The model under review builds one solid part; all positions refer to its coordinate system, in mm. A direction names the side the tool comes from. Round coordinates to 2 decimals unless told otherwise and drop trailing zeros. Loops run counter-clockwise (first coordinate to the right, second up) from the corner with the lowest first, then second, coordinate; pieces in that order, holes last. Notation, with made-up numbers: M 24,11 L 57,11 A25 cw 57,34 Z; hole C 29,83.25 d5. An arc over 180 degrees is marked long. One line per question, with ' | ' between items.
from build123d import *

# Parameters (mm, degrees)
SKETCH3_W                 = 4.35
SKETCH3_H                 = 3.42
SKETCH_PATTERN1_START     = -2.691666667
SKETCH_PATTERN1_OUTLINE_R = 4.35
SKETCH_PATTERN1_DEPTH     = 3.42
SKETCH14_R                = 4.35
CUT_EXTRUDE5_DEPTH        = 0.4275
SKETCH17_OUTSIDE_W        = 88.114
SKETCH17_OUTSIDE_H        = 88.114
SKETCH17_OUTSIDE_R        = 3.768125
CUT_EXTRUDE8_DEPTH        = 9.955029662
CUT_EXTRUDE8_DRAFT        = -75
SKETCH18_OUTSIDE_W        = 82.758
SKETCH18_OUTSIDE_H        = 82.758
SKETCH18_OUTSIDE_R        = 3.768125
CUT_EXTRUDE9_DEPTH        = 9.237544301
CUT_EXTRUDE9_DRAFT        = -75
SKETCH19_OUTSIDE_W        = 93.34
SKETCH19_OUTSIDE_H        = 93.34
SKETCH19_OUTSIDE_R        = 3.768125
CUT_EXTRUDE10_DEPTH       = 10.655226708
CUT_EXTRUDE10_DRAFT       = -75
SKETCH7_R                 = 3
CUT_EXTRUDE1_DEPTH        = 12.317906167
CHAMFER1_SIZE             = 0.158
FILLET2_R                 = 0.1305


# Read off the part's stored shape, not the designer's step: Sketch-Pattern1
with BuildPart() as part:
    # Sketch3 → Revolve1 (revolve)
    with BuildSketch(Plane.XY):
        with Locations((2.175, 3.04)):
            Rectangle(SKETCH3_W, SKETCH3_H)
    revolve(axis=Axis((0, 1.33, 0), (0, 1, 0)))

    # Sketch14 → Cut-Extrude5 (cut)
    with BuildSketch(Plane.XZ.offset(-1.33)):
        Circle(SKETCH14_R)
    extrude(amount=-CUT_EXTRUDE5_DEPTH, mode=Mode.SUBTRACT)


with BuildPart() as body_2:
    # Sketch6 → Revolve2 (revolve)
    with BuildSketch(Plane.XY):
        Polygon((3.7525, 0.728333333), (3.7525, -2.691666667), (3.7525, -3.720833333), (3.95, -3.720833333), (3.95, -4.75), (0, -4.75), (0, 1.7575), (3.7525, 1.7575), align=None)
    revolve(axis=Axis((0, -4.75, 0), (0, 1, 0)))


with BuildPart() as body_3:
    # Sketch-Pattern1 outline → Sketch-Pattern1 (new body)
    with BuildSketch(Plane(origin=(0, 0, 0), x_dir=(1, 0, 0), z_dir=(0, 1, 0)).offset(SKETCH_PATTERN1_START)):
        Circle(SKETCH_PATTERN1_OUTLINE_R)
    extrude(amount=SKETCH_PATTERN1_DEPTH)


with BuildPart() as body_4:
    # Mirror3: mirrored copy
    add(body_3.part.mirror(Plane.XY))


with BuildPart() as cut_extrude8_tool:
    # Sketch17 outside → Cut-Extrude8 (with draft: the straight prism first)
    with BuildSketch(Plane.XZ.offset(-1.7575)):
        Rectangle(SKETCH17_OUTSIDE_W, SKETCH17_OUTSIDE_H)
        Circle(SKETCH17_OUTSIDE_R, mode=Mode.SUBTRACT)
    extrude(amount=-CUT_EXTRUDE8_DEPTH)
    # Cut-Extrude8: the draft: its side faces are tilted about the plane it starts from
    cut_extrude8_sides = [cut_extrude8_tool.faces().sort_by_distance(p)[0] for p in [
        (0, 6.735014831, -44.057),
        (44.057, 6.735014831, 0),
        (0, 6.735014831, 44.057),
        (-44.057, 6.735014831, 0),
        (-3.768125, 6.735014831, 0),
    ]]
    draft(cut_extrude8_sides, Plane.XZ.offset(-1.7575), CUT_EXTRUDE8_DRAFT)


with BuildPart() as part_1:
    add(part.part)

    # Cut-Extrude8: cut by cut_extrude8_tool
    add(cut_extrude8_tool.part, mode=Mode.SUBTRACT)


with BuildPart() as cut_extrude9_tool:
    # Sketch18 outside → Cut-Extrude9 (with draft: the straight prism first)
    with BuildSketch(Plane(origin=(0, 0.728333333, 0), x_dir=(1, 0, 0), z_dir=(0, 1, 0))):
        Rectangle(SKETCH18_OUTSIDE_W, SKETCH18_OUTSIDE_H)
        Circle(SKETCH18_OUTSIDE_R, mode=Mode.SUBTRACT)
    extrude(amount=-CUT_EXTRUDE9_DEPTH)
    # Cut-Extrude9: the draft: its side faces are tilted about the plane it starts from
    cut_extrude9_sides = [cut_extrude9_tool.faces().sort_by_distance(p)[0] for p in [
        (0, -3.890438817, 41.379),
        (41.379, -3.890438817, 0),
        (0, -3.890438817, -41.379),
        (-41.379, -3.890438817, 0),
        (-3.768125, -3.890438817, 0),
    ]]
    draft(cut_extrude9_sides, Plane(origin=(0, 0.728333333, 0), x_dir=(1, 0, 0), z_dir=(0, 1, 0)), CUT_EXTRUDE9_DRAFT)


with BuildPart() as body_4_1:
    add(body_4.part)

    # Cut-Extrude9: cut by cut_extrude9_tool
    add(cut_extrude9_tool.part, mode=Mode.SUBTRACT)


with BuildPart() as cut_extrude10_tool:
    # Sketch19 outside → Cut-Extrude10 (with draft: the straight prism first)
    with BuildSketch(Plane.XZ.offset(2.691666667)):
        Rectangle(SKETCH19_OUTSIDE_W, SKETCH19_OUTSIDE_H)
        Circle(SKETCH19_OUTSIDE_R, mode=Mode.SUBTRACT)
    extrude(amount=-CUT_EXTRUDE10_DEPTH)
    # Cut-Extrude10: the draft: its side faces are tilted about the plane it starts from
    cut_extrude10_sides = [cut_extrude10_tool.faces().sort_by_distance(p)[0] for p in [
        (0, 2.635946687, -46.67),
        (46.67, 2.635946687, 0),
        (0, 2.635946687, 46.67),
        (-46.67, 2.635946687, 0),
        (-3.768125, 2.635946687, 0),
    ]]
    draft(cut_extrude10_sides, Plane.XZ.offset(2.691666667), CUT_EXTRUDE10_DRAFT)


with BuildPart() as body_4_2:
    add(body_4_1.part)

    # Cut-Extrude10: cut by cut_extrude10_tool
    add(cut_extrude10_tool.part, mode=Mode.SUBTRACT)


with BuildPart() as cut_extrude1_tool:
    # Sketch7 → Cut-Extrude1 (new, through all)
    with BuildSketch(Plane(origin=(0, 4.75, 0), x_dir=(1, 0, 0), z_dir=(0, 1, 0))):
        with Locations(Location((0, 0, 0), (0, 0, 180))):
            Circle(SKETCH7_R)
    extrude(amount=-CUT_EXTRUDE1_DEPTH)


with BuildPart() as part_2:
    add(part_1.part)

    # Cut-Extrude1: cut by cut_extrude1_tool
    add(cut_extrude1_tool.part, mode=Mode.SUBTRACT)


with BuildPart() as body_2_1:
    add(body_2.part)

    # Cut-Extrude1: cut by cut_extrude1_tool
    add(cut_extrude1_tool.part, mode=Mode.SUBTRACT)


with BuildPart() as body_4_3:
    add(body_4_2.part)

    # Cut-Extrude1: cut by cut_extrude1_tool
    add(cut_extrude1_tool.part, mode=Mode.SUBTRACT)


with BuildPart() as part_3:
    add(part_2.part)

    # Combine1: union body 4, body 2
    add(body_4_3.part)
    add(body_2_1.part)

    # Chamfer1
    chamfer1_edges = [part_3.edges().sort_by_distance(p)[0] for p in [
        (-3.95, -3.720833333, 0),
        (-3.95, -4.75, 0),
    ]]
    chamfer(chamfer1_edges, length=CHAMFER1_SIZE)

    # Fillet2
    # the kernel refuses this fillet: 0.1305 mm, written as the material it adds along each edge
    with BuildSketch(Plane(origin=(0, 1.7575, 0), x_dir=(1, 0, 0), z_dir=(0, 0, 1))) as fillet2_piece_1:
        with BuildLine():
            CenterArc((3.883, -0.061919176), FILLET2_R, 151.674733073, 28.325266927)
            Line((3.7525, -0.061919176), (3.74989, -0.061919176))
            Line((3.74989, -0.061919176), (3.74989, 0))
            Line((3.74989, 0), (3.7525, 0.00261))
            ThreePointArc((3.7525, 0.00261), (3.7603125, 0.00261), (3.7658275, 0.001238384))
            Line((3.7658275, 0.001238384), (3.768125, 0))
        make_face()
    revolve(axis=Axis((0, 1.7575, 0), (0, 1, 0)))
    with BuildSketch(Plane(origin=(0, -2.691666667, 0), x_dir=(1, 0, 0), z_dir=(0, 0, -1))) as fillet2_piece_2:
        with BuildLine():
            CenterArc((3.883, 0.061919176), FILLET2_R, 180, 28.325266927)
            Line((3.768125, 0), (3.7658275, -0.001238384))
            ThreePointArc((3.7658275, -0.001238384), (3.7603125, -0.00261), (3.7525, -0.00261))
            Line((3.7525, -0.00261), (3.74989, 0))
            Line((3.74989, 0), (3.74989, 0.061919176))
            Line((3.74989, 0.061919176), (3.7525, 0.061919176))
        make_face()
    revolve(axis=Axis((0, -2.691666667, 0), (0, -1, 0)))
    with BuildSketch(Plane(origin=(0, -3.720833333, 0), x_dir=(1, 0, 0), z_dir=(0, 0, 1))) as fillet2_piece_3:
        with BuildLine():
            CenterArc((3.883, 0.093537426), FILLET2_R, 180, 45.78777852)
            Line((3.7525, 0.093537426), (3.74989, 0.093537426))
            Line((3.74989, 0.093537426), (3.74989, 0))
            Line((3.74989, 0), (3.7525, -0.00261))
            ThreePointArc((3.7525, -0.00261), (3.77225, -0.00261), (3.79018, -0.001870749))
            Line((3.79018, -0.001870749), (3.792, 0))
        make_face()
    revolve(axis=Axis((0, -3.720833333, 0), (0, 1, 0)))
    with BuildSketch(Plane(origin=(0, 0.728333333, 0), x_dir=(1, 0, 0), z_dir=(0, 0, -1))) as fillet2_piece_4:
        with BuildLine():
            CenterArc((3.883, -0.061919176), FILLET2_R, 151.674733073, 28.325266927)
            Line((3.768125, 0), (3.7658275, 0.001238383))
            ThreePointArc((3.7658275, 0.001238383), (3.7603125, 0.00261), (3.7525, 0.00261))
            Line((3.7525, 0.00261), (3.74989, 0))
            Line((3.74989, 0), (3.74989, -0.061919176))
            Line((3.74989, -0.061919176), (3.7525, -0.061919176))
        make_face()
    revolve(axis=Axis((0, 0.728333333, 0), (0, -1, 0)))


solid = part_3.part
1) For line 1 (Z direction, x = 0, y = -0.5); line 2 (Y direction, x = -2.75, z = 2.75); line 3 (Z direction, x = 1, y = -0.5), list the stretches that pass through material, from the lowest coordinate up.
Output values:
line 1: z = -4.35 to -3, 3 to 4.35 | line 2: y = -4.65 to -3.82, -2.66 to 0.7, 1.79 to 4.75 | line 3: z = -4.23 to -2.83, 2.83 to 4.23
2) Insertion check: P1, Ø4, axis at x = 0, z = -1.5, coming from the -Y side; P2, Ø1.5, axis at x = -2, y = 1, coming from the -Z side; P3, Ø4, axis at y = 1.5, z = -2.5, coming from the -X side; P4, Ø5, axis at y = -2.5, z = -3, coming from the +X side. Each pin has a flat end and moves straight along its axis. Give the tip position at first contact, or say it passes through.
Output values:
P1: stops at y = -4.75 | P2: stops at z = -4.12 | P3: stops at x = -4.32 | P4: stops at x = 4.32
3) Add section D-D on y = 1.25. State the section outline as (x, z) points (1 decimal).
Output values:
outline: C 0,0 d7.5; hole C 0,0 d6
4) Machinability: for faces 1 (the cylindrical face through (-0.943, 3.352, 4.247)), 2 (the cylindrical face through (3.58, -3.18, -1.13)), 3 (the cylindrical face through (-3.135, -4.24, 2.404)), which of the approach directions +Z, -Z, +X, -X, +Y, -Y give a long, thin tool a straight path to every point of the face, cutting with its end or side? Answer none if there is none.
Output values:
face 1: +Y, -Y | face 2: none | face 3: -Y
5) Add section C-C on y = 3.75. State the section outline as (x, z) points, then the cut area to 3 significant figures.
Output values:
outline: C 0,0 d8.7; hole C 0,0 d6 | area: 31.2 mm²
6) Mouldability with a two-part tool opening along Z and no side actions: class faces 4 (the cylindrical face through (3.58, 1.25, -1.13)), 5 (the cylindrical face through (-2.86, 0.07, 0.9)), 6 (the flat face through (3, -4.75, -1)) as +Z half, -Z half, draft (parallel to the pull), parting line (faces both ways), or undercut.
Output values:
face 4: parting line | face 5: undercut | face 6: draft
